Verification items for the finished model (mm, model axes). A direction names the side the tool comes from. Round coordinates to 2 decimals unless told otherwise and drop trailing zeros. Loops run counter-clockwise (first coordinate to the right, second up) from the corner with the lowest first, then second, coordinate; pieces in that order, holes last. Notation, with made-up numbers: M -21.75,-24.75 L 20.25,-24.75 A17 ccw 20.25,-20.75 Z; hole C 88,8.25 d1. An arc over 180 degrees is marked long. Answer as CSV lines item,"result".
```python
from build123d import *

# Parameters (mm, degrees)
SKETCH1_R           = 10
BOSS_EXTRUDE1_DEPTH = 4
BODY_START          = 5
SKETCH2_R           = 10
BODY_HOLE_DEPTH     = 2
SKETCH5_R           = 0.8
SCREW_HOLES_DEPTH   = 5
SKETCH6_R           = 1.25
SCREW_HEADS_DEPTH   = 2
POT_START           = 0.5
POT_INSERT_DEPTH    = 2.5
SKETCH4_R           = 2.75
POT_HOLE_DEPTH      = 5
CUT_REVOLVE6_ANGLE  = 180
CUT_EXTRUDE1_DEPTH  = 14.999999999


with BuildPart() as part:
    # Sketch1 → Boss-Extrude1 (new body)
    with BuildSketch(Plane.XY):
        Circle(SKETCH1_R)
        with BuildLine():
            Line((13.999999999, 10), (-1e-09, 10))
            ThreePointArc((-1e-09, 10), (7.071067811, 7.071067812), (9.999999999, 0))
            ThreePointArc((9.999999999, 0), (7.071067811, -7.071067812), (-1e-09, -10))
            Line((-1e-09, -10), (13.999999999, -10))
            Line((13.999999999, -10), (13.999999999, 10))
        make_face()
    extrude(amount=BOSS_EXTRUDE1_DEPTH)

    # Sketch2 → Body Hole (cut)
    with BuildSketch(Plane.XY.offset(BODY_START)):
        Circle(SKETCH2_R)
        with BuildLine():
            Line((9.999999999, 10), (-1e-09, 10))
            ThreePointArc((-1e-09, 10), (7.071067811, 7.071067812), (9.999999999, 0))
            Line((9.999999999, 0), (9.999999999, 10))
        make_face()
        with BuildLine():
            Line((9.999999999, -10), (9.999999999, 0))
            ThreePointArc((9.999999999, 0), (7.071067811, -7.071067812), (-1e-09, -10))
            Line((-1e-09, -10), (9.999999999, -10))
        make_face()
    extrude(amount=-BODY_HOLE_DEPTH, mode=Mode.SUBTRACT)

    # Sketch5 → Screw Holes (cut, through all)
    with BuildSketch(Plane.XY):
        with Locations((11.999999999, 6.25)):
            Circle(SKETCH5_R)
        with Locations((11.999999999, -6.25)):
            Circle(SKETCH5_R)
    extrude(amount=SCREW_HOLES_DEPTH, mode=Mode.SUBTRACT)

    # Sketch6 → Screw Heads (cut)
    with BuildSketch(Plane.XY):
        with Locations((11.999999999, -6.25)):
            Circle(SKETCH6_R)
    extrude(amount=SCREW_HEADS_DEPTH, mode=Mode.SUBTRACT)

    # Sketch3 → Pot Insert (cut)
    with BuildSketch(Plane(origin=(28.28760271, 0, 0), x_dir=(1, 0, 0), z_dir=(0, 0, 1)).offset(POT_START)):
        Polygon((-35.287602709, 0), (-35.287602709, -1.5), (-33.787602709, -1.5), (-32.287602709, -4.5), (-32.287602709, -5.5), (-28.287602709, -5.5), (-24.037602709, -5.5), (-24.037602709, -4.5), (-18.787602709, -4.5), (-18.787602709, 0), (-18.787602709, 4.5), (-24.037602709, 4.5), (-24.037602709, 5.5), (-28.287602709, 5.5), (-32.287602709, 5.5), (-32.287602709, 4.5), (-33.787602709, 1.5), (-35.287602709, 1.5), align=None)
    extrude(amount=POT_INSERT_DEPTH, mode=Mode.SUBTRACT)

    # Sketch4 → Pot Hole (cut, through all)
    with BuildSketch(Plane.XY):
        Circle(SKETCH4_R)
    extrude(amount=POT_HOLE_DEPTH, mode=Mode.SUBTRACT)

    # Sketch11 → Cut-Revolve6 (revolve, cut)
    with BuildSketch(Plane(origin=(0, 0, 0), x_dir=(0, 0, -1), z_dir=(1, 0, 0))):
        with BuildLine():
            Line((1.680646386, 2.75), (2, 2.75))
            Line((2, 2.75), (2, 12))
            Line((2, 12), (-10, 12))
            ThreePointArc((-10, 12), (-2.550167787, 9.407443861), (1.680646386, 2.75))
        make_face()
    revolve(axis=Axis((0, 0, 0), (0, 0, 1)), revolution_arc=CUT_REVOLVE6_ANGLE, mode=Mode.SUBTRACT)

    # Sketch13 → Cut-Extrude1 (cut, through all)
    with BuildSketch(Plane(origin=(0, 0, 0), x_dir=(0, 0, -1), z_dir=(1, 0, 0))):
        with BuildLine():
            Line((2, 12), (-10, 12))
            ThreePointArc((-10, 12), (-1.514718626, 8.485281374), (2, 0))
            Line((2, 0), (2, 12))
        make_face()
        with BuildLine():
            Line((2, 0), (2, -12))
            Line((2, -12), (-10, -12))
            ThreePointArc((-10, -12), (-1.514718626, -8.485281374), (2, 0))
        make_face()
    extrude(amount=CUT_EXTRUDE1_DEPTH, mode=Mode.SUBTRACT)


solid = part.part
```
1) Material ranges on probe 1 along X at (y, z) = (-1.25, 3.1); probe 2 along Y at (x, z) = (12, 2.6); probe 3 along Y at (x, z) = (3.25, 2.5), recorded low to high.
Here are the results:
probe 1,"x = 10 to 14"
probe 2,"y = -9.45 to -7.05, -5.45 to 5.45, 7.05 to 9.45"
probe 3,"y = -9.37 to -5.5, 5.5 to 9.37"
2) Set-up check for faces 1 (the flat face through (-4, 5, 2)), 2 (the flat face through (13, -6, 2)), 3 (the flat face through (-4.4, -4.2, 3)): record each of +Z, -Z, +X, -X, +Y, -Y from which the full face is reachable in a straight line by a thin tool's end or side.
Here are the results:
face 1,"+Z"
face 2,"-Z"
face 3,"+Z, -X, +Y, -Y"
3) Go/stop test with flat-tipped pins: pin 1 (1.5 mm diameter, centred on y = -5, z = 2, fed in from -X); pin 2 (0.8 mm diameter, centred on x = -6.5, z = 2.5, fed in from -Y); pin 3 (0.5 mm diameter, centred on y = -5, z = 1.5, fed in from -X). Record where each tip stops, or that it passes through.
Here are the results:
pin 1,"stops at x = -8.28"
pin 2,"stops at y = -7.3"
pin 3,"stops at x = -7.18"
4) Section check C-C (z = 2.5). State how many separate pieces and enclosed holes the cut face has, plus the area to 3 significant figures.
Here are the results:
separate pieces,"1"
enclosed holes,"3"
area,"245 mm^2"
5) Section check A-A (y = 0). Record the cut outline in (x, z), plus the area to 3 significant figures.
Here are the results:
outline,"M -9.75,3 A12 ccw -6.63,0 L -2.75,0 L -2.75,0.5 L -7,0.5 L -7,3 Z; M 2.75,0 L 14,0 L 14,4 L 10,4 L 10,3 L 9.5,3 L 9.5,0.5 L 2.75,0.5 Z"
area,"27.1 mm^2"
6) Section check D-D (x = -0.5). Record the cut outline in (y, z), plus the area to 3 significant figures.
Here are the results:
outline,"M -9.73,3 A11.99 ccw -6.61,0 L -2.7,0 L -2.7,0.5 L -5.5,0.5 L -5.5,3 Z; M 2.7,0 L 6.61,0 A11.99 ccw 9.73,3 L 5.5,3 L 5.5,0.5 L 2.7,0.5 Z"
area,"20.0 mm^2"
7) Draft check along X on faces 4 (the flat face through (4, 0, 0)), 5 (the flat face through (4.25, -5, 2)). Enter one of: +X half, -X half, draft (parallel to the pull), parting line (faces both ways), or undercut.
Here are the results:
face 4,"draft"
face 5,"undercut"
8) Section check B-B (x = 8.75). Record the cut outline in (y, z).
Here are the results:
outline,"M -9.75,3 A12 ccw -6.63,0 L 6.63,0 A12 ccw 9.75,3 L 4.5,3 L 4.5,0.5 L -4.5,0.5 L -4.5,3 Z"
